Model file for the job. Use its own axes, mm. A direction names the side the tool comes from. Coordinates: 2 decimals unless noted, no trailing zeros. Loops run counter-clockwise (first coordinate to the right, second up) from the corner with the lowest first, then second, coordinate; pieces in that order, holes last. Notation, with made-up numbers: (80, 60.25) - (94, 60.25) arc R21 cw to (94, 93.25) - close; hole circle Ø11 at (59.5, -28.75). An arc over 180 degrees is marked (long way). Write each question's results on one line, items separated by ' | '. Start each with the question number.
```python
from build123d import *

# Parameters (mm, degrees)
SKETCH1_R           = 8
BOSS_EXTRUDE1_DEPTH = 3
SKETCH2_W           = 17
SKETCH2_H           = 3
BOSS_EXTRUDE2_DEPTH = 17
SKETCH3_W           = 45
SKETCH3_H           = 3
BOSS_EXTRUDE3_DEPTH = 9.2
BOSS_EXTRUDE4_REACH = 41.571
SKETCH4_W           = 5.3
SKETCH4_H           = 3
SKETCH6_W           = 45
SKETCH6_H           = 5.3
BOSS_EXTRUDE5_DEPTH = 9.2
SKETCH7_W           = 17
SKETCH7_H           = 3
BOSS_EXTRUDE6_DEPTH = 11.7
SKETCH8_R           = 1.525
CUT_EXTRUDE1_DEPTH  = 44.180319591
CHAMFER1_SIZE       = 5
FILLET1_R           = 5
SKETCH9_R           = 1.5
SKETCH9_R_2         = 1.525
CUT_EXTRUDE2_DEPTH  = 44.180319591
FILLET2_R           = 2


with BuildPart() as part:
    # Sketch1 → Boss-Extrude1 (new body)
    with BuildSketch(Plane.XY):
        with BuildLine():
            Line((-17.5, -10.5), (17.5, -10.5))
            ThreePointArc((17.5, -10.5), (21.035533906, -9.035533906), (22.5, -5.5))
            Line((22.5, -5.5), (22.5, 10.5))
            Line((22.5, 10.5), (22.5, 13))
            Line((22.5, 13), (-22.5, 13))
            Line((-22.5, 13), (-22.5, 10.5))
            Line((-22.5, 10.5), (-22.5, -5.5))
            ThreePointArc((-22.5, -5.5), (-21.035533906, -9.035533906), (-17.5, -10.5))
        make_face()
        with Locations((13, -0.5)):
            Circle(SKETCH1_R, mode=Mode.SUBTRACT)
        with Locations((-13, -0.5)):
            Circle(SKETCH1_R, mode=Mode.SUBTRACT)
    extrude(amount=BOSS_EXTRUDE1_DEPTH)

    # Sketch2 → Boss-Extrude2 (add)
    with BuildSketch(Plane(origin=(0, 0, 0), x_dir=(-1, 0, 0), z_dir=(0, 0, -1))):
        with Locations((-14, 11.5)):
            Rectangle(SKETCH2_W, SKETCH2_H)
        with Locations((14, 11.5)):
            Rectangle(SKETCH2_W, SKETCH2_H)
    extrude(amount=BOSS_EXTRUDE2_DEPTH)

    # Sketch3 → Boss-Extrude3 (add)
    with BuildSketch(Plane(origin=(0, 13, 0), x_dir=(1, 0, 0), z_dir=(0, 1, 0))):
        with Locations((0, -1.5)):
            Rectangle(SKETCH3_W, SKETCH3_H)
    extrude(amount=BOSS_EXTRUDE3_DEPTH)

    # Sketch4 → Boss-Extrude4 (add, up to next)
    with BuildSketch(Plane(origin=(-5.5, 0, 0), x_dir=(0, 0, -1), z_dir=(1, 0, 0)), mode=Mode.PRIVATE) as boss_extrude4_sk1:
        with Locations((2.65, 11.5)):
            Rectangle(SKETCH4_W, SKETCH4_H)
    boss_extrude4_tool1 = extrude(boss_extrude4_sk1.sketch, amount=BOSS_EXTRUDE4_REACH, mode=Mode.PRIVATE) - part.part
    add(boss_extrude4_tool1.solids().sort_by_distance((-5.5, 11.5, -2.65))[0])

    # Sketch6 → Boss-Extrude5 (add)
    with BuildSketch(Plane(origin=(0, 13, 0), x_dir=(1, 0, 0), z_dir=(0, 1, 0))):
        with Locations((0, 2.65)):
            Rectangle(SKETCH6_W, SKETCH6_H)
    extrude(amount=BOSS_EXTRUDE5_DEPTH)

    # Sketch7 → Boss-Extrude6 (add, through all)
    with BuildSketch(Plane(origin=(0, 0, -5.3), x_dir=(-1, 0, 0), z_dir=(0, 0, -1))):
        with Locations((-14, 20.7)):
            Rectangle(SKETCH7_W, SKETCH7_H)
        with Locations((14, 20.7)):
            Rectangle(SKETCH7_W, SKETCH7_H)
    extrude(amount=BOSS_EXTRUDE6_DEPTH)

    # Sketch8 → Cut-Extrude1 (cut, through all)
    with BuildSketch(Plane(origin=(0, 22.2, 0), x_dir=(1, 0, 0), z_dir=(0, 1, 0))):
        with Locations(Location((14, 14, 0), (0, 0, 270))):
            Circle(SKETCH8_R)
        with Locations(Location((-14, 14, 0), (0, 0, 270))):
            Circle(SKETCH8_R)
    extrude(amount=-CUT_EXTRUDE1_DEPTH, mode=Mode.SUBTRACT)

    # Chamfer1
    chamfer1_edges = [part.edges().sort_by_distance(p)[0] for p in [
        (0, 22.2, 3),
    ]]
    chamfer(chamfer1_edges, length=CHAMFER1_SIZE)

    # Fillet1
    fillet1_edges = [part.edges().sort_by_distance(p)[0] for p in [
        (22.5, 20.7, -17),
        (5.5, 20.7, -17),
        (-22.5, 20.7, -17),
        (-5.5, 20.7, -17),
        (5.5, 11.5, -17),
        (22.5, 11.5, -17),
        (-5.5, 11.5, -17),
        (-22.5, 11.5, -17),
    ]]
    fillet(fillet1_edges, radius=FILLET1_R)

    # Sketch9 → Cut-Extrude2 (cut, through all)
    # profile 1 of 2: a face of its own
    with BuildSketch(Plane(origin=(0, 22.2, 0), x_dir=(1, 0, 0), z_dir=(0, 1, 0))):
        with Locations(Location((-18.8, 14, 0), (0, 0, 270))):
            Circle(SKETCH9_R)
    # profile 2 of 2: a face of its own
    with BuildSketch(Plane(origin=(0, 22.2, 0), x_dir=(1, 0, 0), z_dir=(0, 1, 0))):
        with BuildLine():
            Line((-5.5, 10.41), (-12.349475382, 10.41))
            Line((-12.349475382, 10.41), (-12.849475382, 10.41))
            ThreePointArc((-12.849475382, 10.41), (-15.194497894, 11.45415993), (-16.156081538, 13.834235021))
            Line((-16.156081538, 13.834235021), (-16.156081538, 17))
            Line((-16.156081538, 17), (-10.5, 17))
            ThreePointArc((-10.5, 17), (-6.964466094, 15.535533906), (-5.5, 12))
            Line((-5.5, 12), (-5.5, 10.41))
        make_face()
        with Locations((-14, 14)):
            Circle(SKETCH9_R_2, mode=Mode.SUBTRACT)
    extrude(amount=-CUT_EXTRUDE2_DEPTH, mode=Mode.SUBTRACT)

    # Fillet2
    fillet2_edges = [part.edges().sort_by_distance(p)[0] for p in [
        (-16.156081538, 20.7, -17),
        (-16.156081538, 11.5, -17),
    ]]
    fillet(fillet2_edges, radius=FILLET2_R)


solid = part.part
```
Q1. Which spindle directions (+Z, -Z, +X, -X, +Y, -Y) get a long thin tool onto all of the face, cutting with end or side? Do faces 4 (the cylindrical face through (12.647, 20.721, -13.296)), 5 (the flat face through (-16, 13, -8)), 6 (the flat face through (-5.5, 21, -8)). Say none if no direction does.
Q2. Mould opens along Z. For faces 1 (the flat face through (0, 0, 0)), 2 (the flat face through (-22.5, 11, -3)), 3 (the cylindrical face through (-17.79, 20.72, -15.11)) say: +Z half, -Z half, draft (parallel to the pull), parting line (faces both ways), or undercut.
Q3. Drill centre lines: L1, parallel to Y at x = 18, z = -13.25; L2, parallel to X at y = 11.15, z = -14 (3 decimals); L3, parallel to Z at x = -11, y = 16. Where is each one in solid material? Low to high. Write a range as from..to.
Q4. Pin check, flat tips, straight feed: pin 1 (0.5 mm diameter, centred on y = 20, z = -14, fed in from +X); pin 2 (14.5 mm diameter, centred on x = 13, y = -0.5, fed in from +Z); pin 3 (4 mm diameter, centred on y = 17.5, z = -15, fed in from +X); pin 4 (10 mm diameter, centred on y = 14, z = -14.5, fed in from -X). Stop position of each tip, or through.
Q5. Cut at D-D (x = 8). List the corners of the cut face in (y, z) (3 decimals), and give its area (3 significant figures).
Q6. Cut at B-B (x = 13). List the corners of the cut face in (y, z), and give its area (3 significant figures).
Q7. Cut at A-A (y = -0.5). List the corners of the cut face in (x, z), and give its area (3 significant figures).
Q8. Cut at C-C (y = 6). List the corners of the cut face in (x, z), and give its area (3 significant figures).
Check result:
1) face 4: +Y, -Y | face 5: -Z, +X, -X | face 6: -Z, +Y, -Y
2) face 1: -Z half | face 2: draft | face 3: undercut
3) L1: 10..13, 19.2..22.2 | L2: -22.083..-20.3, -17.3..-16.156, 5.917..12.475, 15.525..22.083 | L3: -5.3..3
4) pin 1: x = 22.18 | pin 2: through | pin 3: x = 22.11 | pin 4: x = -22.5
5) outline: (-10.5, 0) - (-6.745, 0) - (-6.745, 3) - (-10.5, 3) - close; (5.745, 0) - (10, 0) - (10, -16.33) - (13, -16.33) - (13, -5.3) - (19.2, -5.3) - (19.2, -16.33) - (22.2, -16.33) - (22.2, -2) - (17.2, 3) - (5.745, 3) - close | area: 179 mm²
6) outline: (-10.5, 0) - (-8.5, 0) - (-8.5, 3) - (-10.5, 3) - close; (7.5, 0) - (10, 0) - (10, -12.85) - (13, -12.85) - (13, -5.3) - (19.2, -5.3) - (19.2, -12.85) - (22.2, -12.85) - (22.2, -2) - (17.2, 3) - (7.5, 3) - close; (10, -17) - (13, -17) - (13, -15.15) - (10, -15.15) - close; (19.2, -17) - (22.2, -17) - (22.2, -15.15) - (19.2, -15.15) - close | area: 159 mm²
7) outline: (-22.5, 0) - (-21, 0) - (-21, 3) - (-22.5, 3) - close; (-5, 0) - (5, 0) - (5, 3) - (-5, 3) - close; (21, 0) - (22.5, 0) - (22.5, 3) - (21, 3) - close | area: 39.0 mm²
8) outline: (-22.5, 0) - (-17.66, 0) - (-17.66, 3) - (-22.5, 3) - close; (-8.34, 0) - (8.34, 0) - (8.34, 3) - (-8.34, 3) - close; (17.66, 0) - (22.5, 0) - (22.5, 3) - (17.66, 3) - close | area: 79.0 mm²
